Can you work these out from the model? Positions are in its coordinate system, mm. Round coordinates to 2 decimals unless told otherwise and drop trailing zeros. Order: outer loops, then holes, each group sorted by start corner. A loop starts at its lowest first (then second) coordinate and runs counter-clockwise, first axis right, second up. Notation, with made-up numbers: (29, -17) -> (69, -17) arc R9 cw to (69, -9) -> close; hole circle Ø9 at (25.25, -10). An arc over 180 degrees is marked (long way). One line per item, written item: value.
```python
from build123d import *

# Parameters (mm, degrees)
F0_W     = 100
F0_H     = 25
F1_DEPTH = 4
F4_DEPTH = 4.001
F2_R     = 3
F5_DEPTH = 4.001


with BuildPart() as f1:
    # F0 (on Front) → F1 (new body)
    with BuildSketch(Plane.XZ):
        Rectangle(F0_W, F0_H)
    extrude(amount=F1_DEPTH)

    # F3 (on face) → F4 (cut, through all)
    with BuildSketch(Plane.XZ.offset(4)):
        with BuildLine():
            ThreePointArc((38.027449, 12.5), (49.463037, 0.321938), (38.754359, -12.5))
            Line((38.754359, -12.5), (50, -12.5))
            Line((50, -12.5), (50, 12.5))
            Line((50, 12.5), (38.027449, 12.5))
        make_face()
    extrude(amount=-F4_DEPTH, mode=Mode.SUBTRACT)

    # F2 (on face) → F5 (cut, through all)
    with BuildSketch(Plane.XZ.offset(4)):
        with Locations((37.5, 0)):
            Circle(F2_R)
    extrude(amount=-F5_DEPTH, mode=Mode.SUBTRACT)


solid = f1.part
```
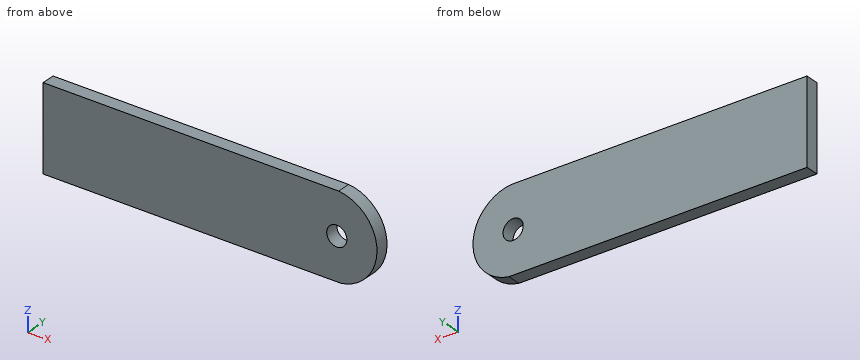
Q1. Please list where these lines run through material, in increasing order: line 1 along Z through (x, y) = (37.5, -1.3); line 2 along Z through (x, y) = (44, -0.95); line 3 along X through (y, z) = (-0.3, -2.25).
Answers below:
line 1: -12.5 to -3, 3 to 12.5
line 2: -10.43 to 10.34
line 3: -50 to 35.52, 39.48 to 49.27
Q2. I want a section at B-B on y = -3.3. List the corners of the cut face in (x, z) for me.
Answers below:
outline: (-50, -12.5) -> (38.75, -12.5) arc R12.6 ccw to (38.03, 12.5) -> (-50, 12.5) -> close; hole circle Ø6 at (37.5, 0)
Q3. I want a section at D-D on z = 8. List the corners of the cut face in (x, y) for me.
Answers below:
outline: (-50, -4) -> (46.57, -4) -> (46.57, 0) -> (-50, 0) -> close
Q4. I want a section at A-A on z = 0. List the corners of the cut face in (x, y) for me, plus the area to 3 significant figures.
Answers below:
outline: (-50, -4) -> (34.5, -4) -> (34.5, 0) -> (-50, 0) -> close; (40.5, -4) -> (49.47, -4) -> (49.47, 0) -> (40.5, 0) -> close
area: 374 mm^2
Q5. I want a section at C-C on z = -8. List the corners of the cut face in (x, y) for me, plus the area to 3 significant figures.
Answers below:
outline: (-50, -4) -> (46.64, -4) -> (46.64, 0) -> (-50, 0) -> close
area: 387 mm^2
